Read the model definition and answer for the solid it produces. Units are mm, in the model's axes. Give positions to 0.01 mm unless a question says otherwise; leave off trailing zeros. Write each loop counter-clockwise with the first axis right and the second up, starting at its lowest first coordinate (ties: lowest second). Pieces come first, ordered by that corner, then holes. Notation, with made-up numbers: M -10.5,-34 L 19.5,-34 A14 ccw 19.5,-24 Z; hole C -22.5,-25 d9. An arc over 180 degrees is marked long. Use a Markdown table: item, result. Add a question column.
Item 1: Consider probe 1 along Z at (x, y) = (0, -2); probe 2 along Z at (x, y) = (-2.5, -2.15); probe 3 along X at (y, z) = (-1.3, 36). Determine where each line is inside the solid, lowest interval first. Write a range as [from, to].
Item 2: Given P1, Ø0.9, axis at y = -1.5, z = 38, coming from the +X side; P2, Ø0.6, axis at x = 20, y = -1, coming from the -Z side; P3, Ø1.5, axis at y = -2, z = -38, coming from the +X side; P4, Ø3, axis at x = 6.91, z = 6.91, coming from the -Y side, each flat-ended and moving along its own axis, determine where each tip first touches the part or whether it passes through.
Item 3: A cutting plane is placed at C-C on x = -32. Determine the outline of the cut face in (y, z), then the cut area to 3 significant figures.
Item 4: A cutting plane is placed at B-B on z = 0. Determine the outline of the cut face in (x, y).
Item 5: A cutting plane is placed at A-A on x = 0. Determine the outline of the cut face in (y, z).
Item 6: A cutting plane is placed at D-D on y = -1.5. Count the separate pieces of the cut face and the enclosed holes in it, then the cut area to 3 significant figures.
from build123d import *

# Parameters (mm, degrees)
F0_R     = 90
F0_R_2   = 1.75
F0_W     = 30
F0_H     = 0.5
F0_R_3   = 3.17
F1_DEPTH = 3


with BuildPart() as f1:
    # F0 (on Front) → F1 (new body)
    with BuildSketch(Plane.XZ):
        Circle(F0_R)
        with BuildLine():
            Line((-29.926763, -82.223104), (-29.755752, -81.753258))
            ThreePointArc((-29.755752, -81.753258), (-18.088317, -85.098841), (-6.068813, -86.788072))
            Line((-6.068813, -86.788072), (-6.103691, -87.286854))
            ThreePointArc((-6.103691, -87.286854), (-18.192273, -85.587915), (-29.926763, -82.223104))
        make_face(mode=Mode.SUBTRACT)
        Polygon((-20.795181, -76.835932), (-20.408811, -76.93946), (-21.702906, -81.769089), (-22.089276, -81.665561), align=None, mode=Mode.SUBTRACT)
        Polygon((-19.5, -25.15), (-20, -25.15), (-20, -15.15), (-20, -13.15), (-19.5, -13.15), (-19.5, -15.15), align=None, mode=Mode.SUBTRACT)
        with Locations((-6.914797, -6.914797)):
            Circle(F0_R_2, mode=Mode.SUBTRACT)
        with BuildLine():
            Line((6.103691, -87.286854), (6.068813, -86.788072))
            ThreePointArc((6.068813, -86.788072), (18.088317, -85.098841), (29.755752, -81.753258))
            Line((29.755752, -81.753258), (29.926763, -82.223104))
            ThreePointArc((29.926763, -82.223104), (18.192273, -85.587915), (6.103691, -87.286854))
        make_face(mode=Mode.SUBTRACT)
        Polygon((22.089276, -81.665561), (21.702906, -81.769089), (20.408811, -76.93946), (20.795181, -76.835932), align=None, mode=Mode.SUBTRACT)
        with BuildLine():
            ThreePointArc((-41.078762, -77.257914), (-45.686982, -74.625396), (-50.127129, -71.718345))
            ThreePointArc((-50.127129, -71.718345), (-50.979425, -70.167154), (-50.266941, -68.546979))
            Line((-50.266941, -68.546979), (-44.332839, -63.567676))
            Line((-44.332839, -63.567676), (-23.722514, -46.27356))
            Line((-23.722514, -46.27356), (-20.714425, -43.749474))
            ThreePointArc((-20.714425, -43.749474), (-20.187384, -43.062621), (-20, -42.217385))
            Line((-20, -42.217385), (-20, -35.15))
            Line((-20, -35.15), (-19.5, -35.15))
            Line((-19.5, -35.15), (-19.5, -42.217385))
            ThreePointArc((-19.5, -42.217385), (-19.734231, -43.27393), (-20.393031, -44.132496))
            Line((-20.393031, -44.132496), (-23.237294, -46.519116))
            ThreePointArc((-23.237294, -46.519116), (0, -52), (23.237294, -46.519116))
            Line((23.237294, -46.519116), (20.393031, -44.132496))
            ThreePointArc((20.393031, -44.132496), (19.734231, -43.27393), (19.5, -42.217385))
            Line((19.5, -42.217385), (19.5, -35.15))
            Line((19.5, -35.15), (20, -35.15))
            Line((20, -35.15), (20, -42.217385))
            ThreePointArc((20, -42.217385), (20.187384, -43.062621), (20.714425, -43.749474))
            Line((20.714425, -43.749474), (23.722514, -46.27356))
            Line((23.722514, -46.27356), (44.332839, -63.567676))
            Line((44.332839, -63.567676), (50.266941, -68.546979))
            ThreePointArc((50.266941, -68.546979), (50.979425, -70.167154), (50.127129, -71.718345))
            ThreePointArc((50.127129, -71.718345), (45.686982, -74.625396), (41.078762, -77.257914))
            Line((41.078762, -77.257914), (40.844026, -76.816441))
            ThreePointArc((40.844026, -76.816441), (45.425914, -74.198965), (49.840688, -71.308525))
            ThreePointArc((49.840688, -71.308525), (50.47991, -70.145133), (49.945547, -68.930001))
            Line((49.945547, -68.930001), (43.906667, -63.862779))
            ThreePointArc((43.906667, -63.862779), (0, -77.5), (-43.906667, -63.862779))
            Line((-43.906667, -63.862779), (-49.945547, -68.930001))
            ThreePointArc((-49.945547, -68.930001), (-50.47991, -70.145133), (-49.840688, -71.308525))
            ThreePointArc((-49.840688, -71.308525), (-45.425914, -74.198965), (-40.844026, -76.816441))
            Line((-40.844026, -76.816441), (-41.078762, -77.257914))
        make_face(mode=Mode.SUBTRACT)
        with Locations((0, -42.217385)):
            Rectangle(F0_W, F0_H, mode=Mode.SUBTRACT)
        Polygon((20, -13.15), (20, -15.15), (20, -25.15), (19.5, -25.15), (19.5, -15.15), (19.5, -13.15), align=None, mode=Mode.SUBTRACT)
        with Locations((6.914797, -6.914797)):
            Circle(F0_R_2, mode=Mode.SUBTRACT)
        with Locations((-6.914797, 6.914797)):
            Circle(F0_R_2, mode=Mode.SUBTRACT)
        Polygon((-19.5, 25.15), (-19.5, 15.15), (-19.5, 13.15), (-20, 13.15), (-20, 15.15), (-20, 25.15), align=None, mode=Mode.SUBTRACT)
        Polygon((-21.702906, 81.769089), (-20.408811, 76.93946), (-20.795181, 76.835932), (-22.089276, 81.665561), align=None, mode=Mode.SUBTRACT)
        with BuildLine():
            Line((-6.103691, 87.286854), (-6.068813, 86.788072))
            ThreePointArc((-6.068813, 86.788072), (-18.088317, 85.098841), (-29.755752, 81.753258))
            Line((-29.755752, 81.753258), (-29.926763, 82.223104))
            ThreePointArc((-29.926763, 82.223104), (-18.192273, 85.587915), (-6.103691, 87.286854))
        make_face(mode=Mode.SUBTRACT)
        Circle(F0_R_3, mode=Mode.SUBTRACT)
        with Locations((6.914797, 6.914797)):
            Circle(F0_R_2, mode=Mode.SUBTRACT)
        Polygon((20, 25.15), (20, 15.15), (20, 13.15), (19.5, 13.15), (19.5, 15.15), (19.5, 25.15), align=None, mode=Mode.SUBTRACT)
        with Locations((0, 42.217385)):
            Rectangle(F0_W, F0_H, mode=Mode.SUBTRACT)
        with BuildLine():
            ThreePointArc((20.714425, 43.749474), (20.187384, 43.062621), (20, 42.217385))
            Line((20, 42.217385), (20, 35.15))
            Line((20, 35.15), (19.5, 35.15))
            Line((19.5, 35.15), (19.5, 42.217385))
            ThreePointArc((19.5, 42.217385), (19.734231, 43.27393), (20.393031, 44.132496))
            Line((20.393031, 44.132496), (23.237294, 46.519116))
            ThreePointArc((23.237294, 46.519116), (0, 52), (-23.237294, 46.519116))
            Line((-23.237294, 46.519116), (-20.393031, 44.132496))
            ThreePointArc((-20.393031, 44.132496), (-19.734231, 43.27393), (-19.5, 42.217385))
            Line((-19.5, 42.217385), (-19.5, 35.15))
            Line((-19.5, 35.15), (-20, 35.15))
            Line((-20, 35.15), (-20, 42.217385))
            ThreePointArc((-20, 42.217385), (-20.187384, 43.062621), (-20.714425, 43.749474))
            Line((-20.714425, 43.749474), (-23.722514, 46.27356))
            Line((-23.722514, 46.27356), (-44.332839, 63.567676))
            Line((-44.332839, 63.567676), (-50.266941, 68.546979))
            ThreePointArc((-50.266941, 68.546979), (-50.979425, 70.167154), (-50.127129, 71.718345))
            ThreePointArc((-50.127129, 71.718345), (-45.686982, 74.625396), (-41.078762, 77.257914))
            Line((-41.078762, 77.257914), (-40.844026, 76.816441))
            ThreePointArc((-40.844026, 76.816441), (-45.425914, 74.198965), (-49.840688, 71.308525))
            ThreePointArc((-49.840688, 71.308525), (-50.47991, 70.145133), (-49.945547, 68.930001))
            Line((-49.945547, 68.930001), (-43.906667, 63.862779))
            ThreePointArc((-43.906667, 63.862779), (0, 77.5), (43.906667, 63.862779))
            Line((43.906667, 63.862779), (49.945547, 68.930001))
            ThreePointArc((49.945547, 68.930001), (50.47991, 70.145133), (49.840688, 71.308525))
            ThreePointArc((49.840688, 71.308525), (45.425914, 74.198965), (40.844026, 76.816441))
            Line((40.844026, 76.816441), (41.078762, 77.257914))
            ThreePointArc((41.078762, 77.257914), (45.686982, 74.625396), (50.127129, 71.718345))
            ThreePointArc((50.127129, 71.718345), (50.979425, 70.167154), (50.266941, 68.546979))
            Line((50.266941, 68.546979), (44.332839, 63.567676))
            Line((44.332839, 63.567676), (23.722514, 46.27356))
            Line((23.722514, 46.27356), (20.714425, 43.749474))
        make_face(mode=Mode.SUBTRACT)
        Polygon((20.795181, 76.835932), (20.408811, 76.93946), (21.702906, 81.769089), (22.089276, 81.665561), align=None, mode=Mode.SUBTRACT)
        with BuildLine():
            Line((29.926763, 82.223104), (29.755752, 81.753258))
            ThreePointArc((29.755752, 81.753258), (18.088317, 85.098841), (6.068813, 86.788072))
            Line((6.068813, 86.788072), (6.103691, 87.286854))
            ThreePointArc((6.103691, 87.286854), (18.192273, 85.587915), (29.926763, 82.223104))
        make_face(mode=Mode.SUBTRACT)
    extrude(amount=F1_DEPTH)


solid = f1.part
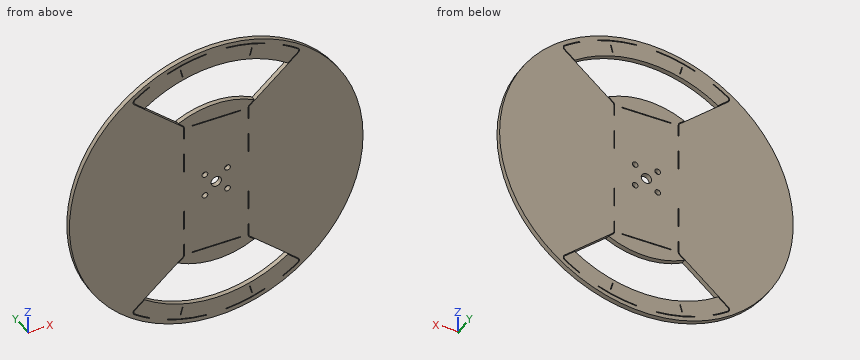
Filled in:
| question | item | result |
|---|---|---|
| 1 | probe 1 | [-90, -77.5], [-52, -42.47], [-41.97, -3.17], [3.17, 41.97], [42.47, 52], [77.5, 90] |
| 1 | probe 2 | [-89.97, -77.46], [-51.94, -42.47], [-41.97, -1.95], [1.95, 41.97], [42.47, 51.94], [77.46, 89.97] |
| 1 | probe 3 | [-82.49, -20], [-19.5, 19.5], [20, 82.49] |
| 2 | P1 | x = 81.79 |
| 2 | P2 | z = -87.82 |
| 2 | P3 | x = 81.93 |
| 2 | P4 | through |
| 3 | outline | M -3,-84.12 L 0,-84.12 L 0,-70.59 L -3,-70.59 Z; M -3,-53.22 L 0,-53.22 L 0,53.22 L -3,53.22 Z; M -3,70.59 L 0,70.59 L 0,84.12 L -3,84.12 Z |
| 3 | area | 401 mm² |
| 4 | outline | M -90,-3 L -3.17,-3 L -3.17,0 L -90,0 Z; M 3.17,-3 L 90,-3 L 90,0 L 3.17,0 Z |
| 5 | outline | M -3,-90 L 0,-90 L 0,-77.5 L -3,-77.5 Z; M -3,-52 L 0,-52 L 0,-42.47 L -3,-42.47 Z; M -3,-41.97 L 0,-41.97 L 0,-3.17 L -3,-3.17 Z; M -3,3.17 L 0,3.17 L 0,41.97 L -3,41.97 Z; M -3,42.47 L 0,42.47 L 0,52 L -3,52 Z; M -3,77.5 L 0,77.5 L 0,90 L -3,90 Z |
| 6 | separate pieces | 1 |
| 6 | enclosed holes | 21 |
| 6 | area | 21,500 mm² |
